Work out the finished part from the listing and answer in its coordinate system (mm). Round coordinates to 2 decimals unless told otherwise and drop trailing zeros. Write each loop counter-clockwise with the first axis right and the second up, starting at its lowest first coordinate (ties: lowest second). Pieces come first, ordered by that corner, then holes.
1. Find section B-B (y = 5). Write down the section's boundary in (x, z).
2. Straight lines are drawn through the part: probe 1 along X at (y, z) = (2.5, 0.55); probe 2 along X at (y, z) = (-14, 0.95); probe 3 along Y at (x, z) = (-3.5, 0.15). For each, find the intervals that lie inside material, in ascending order.
3. Find section C-C (z = 0.75). Count the separate pieces of the cut face and the enclosed holes in it, and give its area (3 significant figures).
4. Find section A-A (x = 0). Write down the section's boundary in (y, z).
5. Find section D-D (x = -4.5). Write down the section's boundary in (y, z), and give its area (3 significant figures).
6. A flat-ended cylindrical pin translates along its axis: pin 1 Ø0.5 at (y, z) = (19.5, 0.5) entering from +X. Find the tip coordinate at first contact, or state that the pin passes through.
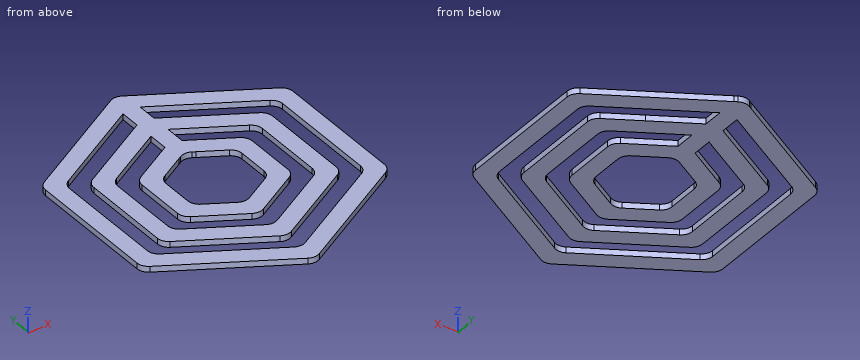
```python
from build123d import *

# Parameters (mm, degrees)
F1_DEPTH = 1
F2_R     = 2


with BuildPart() as f1:
    # F0 (on Top) → F1 (new body)
    with BuildSketch(Plane.XY):
        Polygon((21.650635, -12.5), (21.650635, 12.5), (1.5, 24.133975), (0, 25), (-1.5, 24.133975), (-21.650635, 12.5), (-21.650635, -12.5), (0, -25), align=None)
        Polygon((0, -14.607695), (-12.650635, -7.303848), (-12.650635, 7.303848), (-1.5, 13.74167), (-1.5, 10.277568), (-9.650635, 5.571797), (-9.650635, -5.571797), (0, -11.143594), (9.650635, -5.571797), (9.650635, 5.571797), (1.5, 10.277568), (1.5, 13.74167), (12.650635, 7.303848), (12.650635, -7.303848), align=None, mode=Mode.SUBTRACT)
        Polygon((0, -21.535898), (-18.650635, -10.767949), (-18.650635, 10.767949), (-1.5, 20.669873), (-1.5, 17.205771), (-15.650635, 9.035898), (-15.650635, -9.035898), (0, -18.071797), (15.650635, -9.035898), (15.650635, 9.035898), (9, 12.875644), (1.5, 17.205771), (1.5, 20.669873), (18.650635, 10.767949), (18.650635, -10.767949), align=None, mode=Mode.SUBTRACT)
        Polygon((0, -7.679492), (-6.650635, -3.839746), (-6.650635, 3.839746), (-1.5, 6.813467), (0, 7.679492), (1.5, 6.813467), (6.650635, 3.839746), (6.650635, -3.839746), align=None, mode=Mode.SUBTRACT)
    extrude(amount=F1_DEPTH)

    # F2
    f2_edges = [f1.edges().sort_by_distance(p)[0] for p in [
        (0, 25, 0.5),
        (-21.650635, 12.5, 0.5),
        (-21.650635, -12.5, 0.5),
        (21.650635, 12.5, 0.5),
        (21.650635, -12.5, 0.5),
        (0, -25, 0.5),
        (-18.650635, -10.767949, 0.5),
        (-18.650635, 10.767949, 0.5),
        (18.650635, 10.767949, 0.5),
        (18.650635, -10.767949, 0.5),
        (0, -21.535898, 0.5),
        (0, -14.607695, 0.5),
        (-15.650635, -9.035898, 0.5),
        (-15.650635, 9.035898, 0.5),
        (-9.650635, 5.571797, 0.5),
        (-9.650635, -5.571797, 0.5),
        (0, -11.143594, 0.5),
        (9.650635, -5.571797, 0.5),
        (9.650635, 5.571797, 0.5),
        (12.650635, 7.303848, 0.5),
        (-12.650635, -7.303848, 0.5),
        (-6.650635, 3.839746, 0.5),
        (-6.650635, -3.839746, 0.5),
        (-12.650635, 7.303848, 0.5),
        (0, 7.679492, 0.5),
        (6.650635, 3.839746, 0.5),
        (6.650635, -3.839746, 0.5),
        (0, -7.679492, 0.5),
        (12.650635, -7.303848, 0.5),
        (15.650635, -9.035898, 0.5),
        (0, -18.071797, 0.5),
        (15.650635, 9.035898, 0.5),
    ]]
    fillet(f2_edges, radius=F2_R)


solid = f1.part
```
Worked answers:
1. outline: (-21.65, 0) - (-18.65, 0) - (-18.65, 1) - (-21.65, 1) - close; (-15.65, 0) - (-12.65, 0) - (-12.65, 1) - (-15.65, 1) - close; (-9.56, 0) - (-4.64, 0) - (-4.64, 1) - (-9.56, 1) - close; (4.64, 0) - (9.56, 0) - (9.56, 1) - (4.64, 1) - close; (12.65, 0) - (15.65, 0) - (15.65, 1) - (12.65, 1) - close; (18.65, 0) - (21.65, 0) - (21.65, 1) - (18.65, 1) - close
2. probe 1: x = -21.65 to -18.65, -15.65 to -12.65, -9.65 to -6.65, 6.65 to 9.65, 12.65 to 15.65, 18.65 to 21.65
2. probe 2: x = -19.05 to -13.05, -7.05 to -1.05, 1.05 to 7.05, 13.05 to 19.05
2. probe 3: y = -22.98 to -19.52, -16.05 to -12.59, -9.12 to -5.66, 5.66 to 9.12, 12.59 to 16.05, 19.52 to 22.98
3. separate pieces: 1
3. enclosed holes: 3
3. area: 903 mm2
4. outline: (-24.69, 0) - (-21.23, 0) - (-21.23, 1) - (-24.69, 1) - close; (-17.76, 0) - (-14.3, 0) - (-14.3, 1) - (-17.76, 1) - close; (-10.83, 0) - (-7.37, 0) - (-7.37, 1) - (-10.83, 1) - close; (7.37, 0) - (24.69, 0) - (24.69, 1) - (7.37, 1) - close
5. outline: (-22.4, 0) - (-18.94, 0) - (-18.94, 1) - (-22.4, 1) - close; (-15.47, 0) - (-12.01, 0) - (-12.01, 1) - (-15.47, 1) - close; (-8.55, 0) - (-5.08, 0) - (-5.08, 1) - (-8.55, 1) - close; (5.08, 0) - (8.55, 0) - (8.55, 1) - (5.08, 1) - close; (12.01, 0) - (15.47, 0) - (15.47, 1) - (12.01, 1) - close; (18.94, 0) - (22.4, 0) - (22.4, 1) - (18.94, 1) - close
5. area: 20.8 mm2
6. pin 1: stops at x = 9.96
